Answer from the drawing. Dimensions are ordinates in mm from the lowest x, y and z of the part. A direction names the side the tool comes from. Coordinates: 2 decimals unless noted, no trailing zeros. Write each loop counter-clockwise with the first axis right and the second up, starting at its lowest first coordinate (ties: lowest second). Pieces come first, ordered by that corner, then holes. Notation, with made-up numbers: (-20, 26.25) -> (4, 26.25) arc R28 ccw to (4, 48.25) -> close; hole circle Ø8 at (62.25, 59.5). An arc over 180 degrees is marked (long way). Answer as a JSON object with one key per item and string values. Group by question number.
(1) Which of the six approach directions +Z, -Z, +X, -X, +Y, -Y give full straight-line access (tool end or side, diameter ignored) to the marked faces 1, 2 and 3?
(2) For a pull along Z with two mould halves and no side action, classify the marked faces 4 and 5 as +Z half, -Z half, draft (parallel to the pull), parting line (faces both ways), or undercut.
(3) Find section C-C (x = 385). Give the vertices of the cut face in (y, z).
(4) Straight lines are drawn through the part: L1, parallel to X at y = 2, z = 209.5; L2, parallel to Z at x = 425, y = 41; L3, parallel to Y at x = 396, z = 295. For each, find the intervals that lie inside material, in ascending order.
(5) Find section A-A (z = 164). Give the vertices of the cut face in (x, y).
(6) Find section B-B (x = 214.5). Give the vertices of the cut face in (y, z).
(7) Flat-ended cylindrical pins translate along their axes: P1, Ø6, axis at x = 316, z = 104, coming from the +Y side; P2, Ø1, axis at x = 337, z = 294.5, coming from the -Y side. Find the tip coordinate at first contact, or state that the pin passes through.
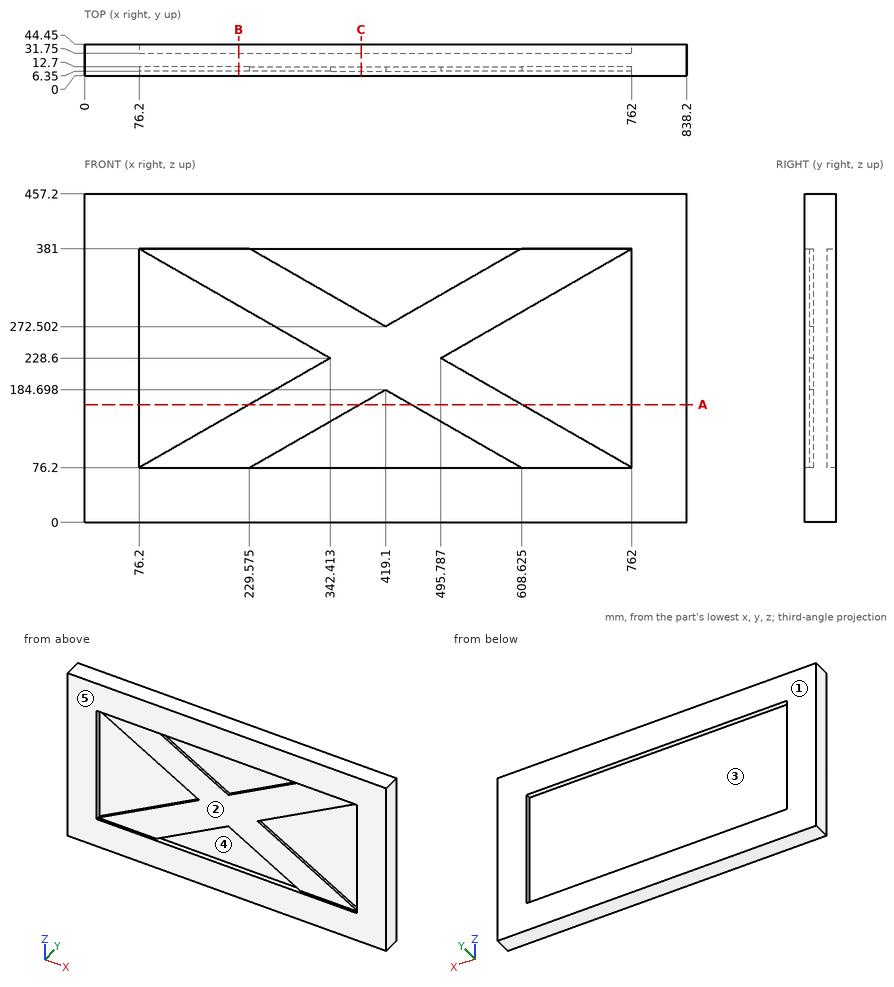
Results below:
{
 "1": {"face 1": "+Z, -Z, +X, -X, +Y", "face 2": "-Y", "face 3": "+Y"},
 "2": {"face 4": "undercut", "face 5": "draft"},
 "3": {"outline": "(0, 0) -> (44.45, 0) -> (44.45, 76.2) -> (31.75, 76.2) -> (31.75, 381) -> (44.45, 381) -> (44.45, 457.2) -> (0, 457.2) -> (0, 381) -> (12.7, 381) -> (12.7, 292.02) -> (6.35, 292.02) -> (6.35, 165.18) -> (12.7, 165.18) -> (12.7, 76.2) -> (0, 76.2) -> close"},
 "4": {"L1": "x = 0 to 76.2, 762 to 838.2", "L2": "z = 0 to 76.2, 381 to 457.2", "L3": "y = 12.7 to 31.75"},
 "5": {"outline": "(0, 0) -> (76.2, 0) -> (76.2, 12.7) -> (229.57, 12.7) -> (229.57, 6.35) -> (382.94, 6.35) -> (382.94, 12.7) -> (455.26, 12.7) -> (455.26, 6.35) -> (608.63, 6.35) -> (608.63, 12.7) -> (762, 12.7) -> (762, 0) -> (838.2, 0) -> (838.2, 44.45) -> (762, 44.45) -> (762, 31.75) -> (76.2, 31.75) -> (76.2, 44.45) -> (0, 44.45) -> close"},
 "6": {"outline": "(0, 0) -> (44.45, 0) -> (44.45, 76.2) -> (31.75, 76.2) -> (31.75, 381) -> (44.45, 381) -> (44.45, 457.2) -> (0, 457.2) -> (0, 381) -> (6.35, 381) -> (6.35, 301.83) -> (12.7, 301.83) -> (12.7, 155.37) -> (6.35, 155.37) -> (6.35, 76.2) -> (0, 76.2) -> close"},
 "7": {"P1": "stops at y = 31.75", "P2": "stops at y = 6.35"}
}
